from build123d import *

# Parameters (mm, degrees)
SKETCH6_R           = 1.5
BOSS_EXTRUDE4_DEPTH = 5
SKETCH8_W           = 44.5
SKETCH8_H           = 44.5
SKETCH8_R           = 1.5
SKETCH8_R_2         = 12.5
BOSS_EXTRUDE5_DEPTH = 50
SKETCH7_W           = 43.5
SKETCH7_H           = 42.5
CUT_EXTRUDE4_DEPTH  = 48.25
BOSS_EXTRUDE6_DEPTH = 1


with BuildPart() as part:
    # Sketch6 → Boss-Extrude4 (new body)
    with BuildSketch(Plane.XY):
        Polygon((-437.521213625, -225.081134847), (-482.021213625, -225.081134847), (-482.021213625, -232.581134847), (-430.021213625, -232.581134847), (-430.021213625, -173.081134847), (-482.021213625, -173.081134847), (-482.021213625, -180.581134847), (-437.521213625, -180.581134847), align=None)
        with Locations((-464.687880625, -228.331134847)):
            Circle(SKETCH6_R, mode=Mode.SUBTRACT)
        with Locations((-447.354547625, -228.331134847)):
            Circle(SKETCH6_R, mode=Mode.SUBTRACT)
        with Locations((-434.271213625, -211.715651861)):
            Circle(SKETCH6_R, mode=Mode.SUBTRACT)
        with Locations((-464.687883625, -176.831134847)):
            Circle(SKETCH6_R, mode=Mode.SUBTRACT)
        with Locations((-434.271213625, -194.382318861)):
            Circle(SKETCH6_R, mode=Mode.SUBTRACT)
        with Locations((-447.354550625, -176.831134847)):
            Circle(SKETCH6_R, mode=Mode.SUBTRACT)
    extrude(amount=BOSS_EXTRUDE4_DEPTH)

    # Sketch8 → Boss-Extrude5 (add)
    with BuildSketch(Plane.XY):
        with Locations((-459.771213625, -202.831134847)):
            Rectangle(SKETCH8_W, SKETCH8_H)
        with Locations((-475.271213625, -218.331134847)):
            Circle(SKETCH8_R, mode=Mode.SUBTRACT)
        with Locations((-444.271213625, -218.331134847)):
            Circle(SKETCH8_R, mode=Mode.SUBTRACT)
        with Locations((-444.271213625, -187.331134847)):
            Circle(SKETCH8_R, mode=Mode.SUBTRACT)
        with Locations((-475.271213625, -187.331134847)):
            Circle(SKETCH8_R, mode=Mode.SUBTRACT)
        with Locations((-460.021213625, -202.581134847)):
            Circle(SKETCH8_R_2, mode=Mode.SUBTRACT)
    extrude(amount=BOSS_EXTRUDE5_DEPTH)

    # Sketch7 → Cut-Extrude4 (cut)
    with BuildSketch(Plane.XY):
        with Locations((-460.271213625, -202.831134847)):
            Rectangle(SKETCH7_W, SKETCH7_H)
    extrude(amount=CUT_EXTRUDE4_DEPTH, mode=Mode.SUBTRACT)

    # Sketch10 → Boss-Extrude6 (add)
    with BuildSketch(Plane.ZY.offset(482.021213625)):
        Polygon((24.125, -181.581134847), (48.25, -224.081134847), (48.25, -181.581134847), align=None)
    extrude(amount=-BOSS_EXTRUDE6_DEPTH)


solid = part.part
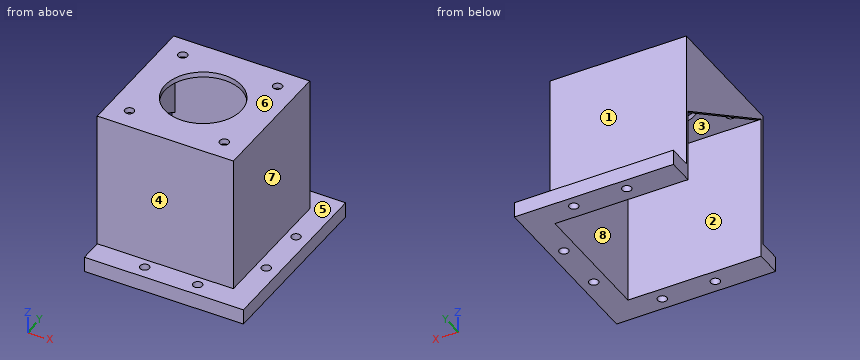
The listing builds one solid part. Answer for the finished solid, in the listing's coordinates (mm). Face numbers are marked on the shaded views. A direction names the side the tool comes from. Round coordinates to 2 decimals unless told otherwise and drop trailing zeros. Loops run counter-clockwise (first coordinate to the right, second up) from the corner with the lowest first, then second, coordinate; pieces in that order, holes last. Notation, with made-up numbers: M 3,30.5 L 45,30.5 A11 ccw 45,44.5 Z; hole C 76.25,-20.75 d9. An arc over 180 degrees is marked long. Write each question's results on one line, items separated by ' | '. Start each with the question number.
1) Find section C-C on x = -440. Write down the section's boundary in (y, z).
2) Straight lines are drawn through the part: probe 1 along Y at (x, z) = (-466, 26); probe 2 along X at (y, z) = (-191, 34.5); probe 3 along Z at (x, y) = (-432, -194). For each, find the intervals that lie inside material, in ascending order.
3) Find section B-B on y = -206.5. Write down the section's boundary in (x, z), plus the area to 3 significant figures.
4) Find section A-A on z = 10.5. Write down the section's boundary in (x, y), plus the area to 4 significant figures.
5) Each of these flat-tipped pins is pushed along its axis until it touches: pin 1 (13.5 mm diameter, centred on y = -192.5, z = 35.5, fed in from +X); pin 2 (5 mm diameter, centred on x = -444.27, y = -218.33, fed in from -Z); pin 3 (5 mm diameter, centred on y = -221, z = 25.5, fed in from -X). Where does it stop, or does it pass through?
6) Find section D-D on x = -458. Write down the section's boundary in (y, z), plus the area to 3 significant figures.
7) Which of the six approach directions +Z, -Z, +X, -X, +Y, -Y give full straight-line access (tool end or side, diameter ignored) to the marked faces 1, 2, 3, 4 and 5?
8) Determine the mould class of the marked faces 6, 7 and 8 for opening direction X: pulls with the +X half, pulls with the -X half, needs draft (parallel to the pull), parting line crosses it, or undercut.
Final values:
1) outline: M -232.58,0 L -224.08,0 L -224.08,48.25 L -181.58,48.25 L -181.58,0 L -173.08,0 L -173.08,5 L -180.58,5 L -180.58,50 L -225.08,50 L -225.08,5 L -232.58,5 Z
2) probe 1: -225.08 to -224.08, -181.58 to -180.58 | probe 2: -482.02 to -481.02, -438.52 to -437.52 | probe 3: 0 to 5
3) outline: M -482.02,38.27 L -481.02,38.27 L -481.02,48.25 L -471.89,48.25 L -471.89,50 L -482.02,50 Z; M -448.15,48.25 L -438.52,48.25 L -438.52,0 L -430.02,0 L -430.02,5 L -437.52,5 L -437.52,50 L -448.15,50 Z | area: 132 mm²
4) outline: M -482.02,-225.08 L -437.52,-225.08 L -437.52,-180.58 L -482.02,-180.58 L -482.02,-181.58 L -438.52,-181.58 L -438.52,-224.08 L -482.02,-224.08 Z | area: 131.5 mm²
5) pin 1: x = -437.52 | pin 2: z = 48.25 | pin 3: x = -438.52
6) outline: M -232.58,0 L -224.08,0 L -224.08,48.25 L -214.92,48.25 L -214.92,50 L -225.08,50 L -225.08,5 L -232.58,5 Z; M -190.25,48.25 L -181.58,48.25 L -181.58,0 L -173.08,0 L -173.08,5 L -180.58,5 L -180.58,50 L -190.25,50 Z | area: 206 mm²
7) face 1: +Z, +X, -X, +Y | face 2: -Z, -X | face 3: -Z | face 4: +Z, +X, -X, -Y | face 5: +Z, +X
8) face 6: needs draft | face 7: pulls with the +X half | face 8: undercut
